For this review, use the dimensioned drawing (mm, ordinates from the lowest corner) and the shaded views. Give positions to 0.01 mm unless a question says otherwise; leave off trailing zeros. Loops run counter-clockwise (first coordinate to the right, second up) from the corner with the lowest first, then second, coordinate; pieces in that order, holes last. Notation, with made-up numbers: M 21.5,80 L 63.5,80 A23 cw 63.5,90 Z; hole C -26,-25.75 d7. An arc over 180 degrees is marked long. Use a Markdown table: item, result. Add a question column.
(1) Add section B-B, the plane y = 30.5. Give the boundary of the cut face in (x, z) (1 decimal), then the cut area to 3 significant figures.
(2) Insertion check: pin 1 Ø5 at (y, z) = (44, 68) entering from -X; pin 2 Ø10 at (y, z) = (14.5, 141.5) entering from -X (1 decimal); pin 3 Ø10 at (y, z) = (6, 19) entering from -X. Each pin has a flat end and moves straight along its axis. Give the tip position at first contact, or say it passes through.
(3) Add section C-C, the plane z = 128. Give the boundary of the cut face in (x, y), then the cut area to 3 significant figures.
(4) For probe 1 along Y at (x, z) = (56.5, 147.5); probe 2 along Y at (x, z) = (107, 66); probe 3 along X at (y, z) = (3, 42.5) (1 decimal), list the stretches that pass through material, from the lowest coordinate up.
(5) Add section D-D, the plane x = 25.5. Give the boundary of the cut face in (y, z) (1 decimal), then the cut area to 3 significant figures.
(6) Draft analysis for pull direction X (two halves, no side actions). For the marked faces 1, 2 and 3, state which applies: pulls with the +X half, pulls with the -X half, needs draft (parallel to the pull), parting line crosses it, or undercut.
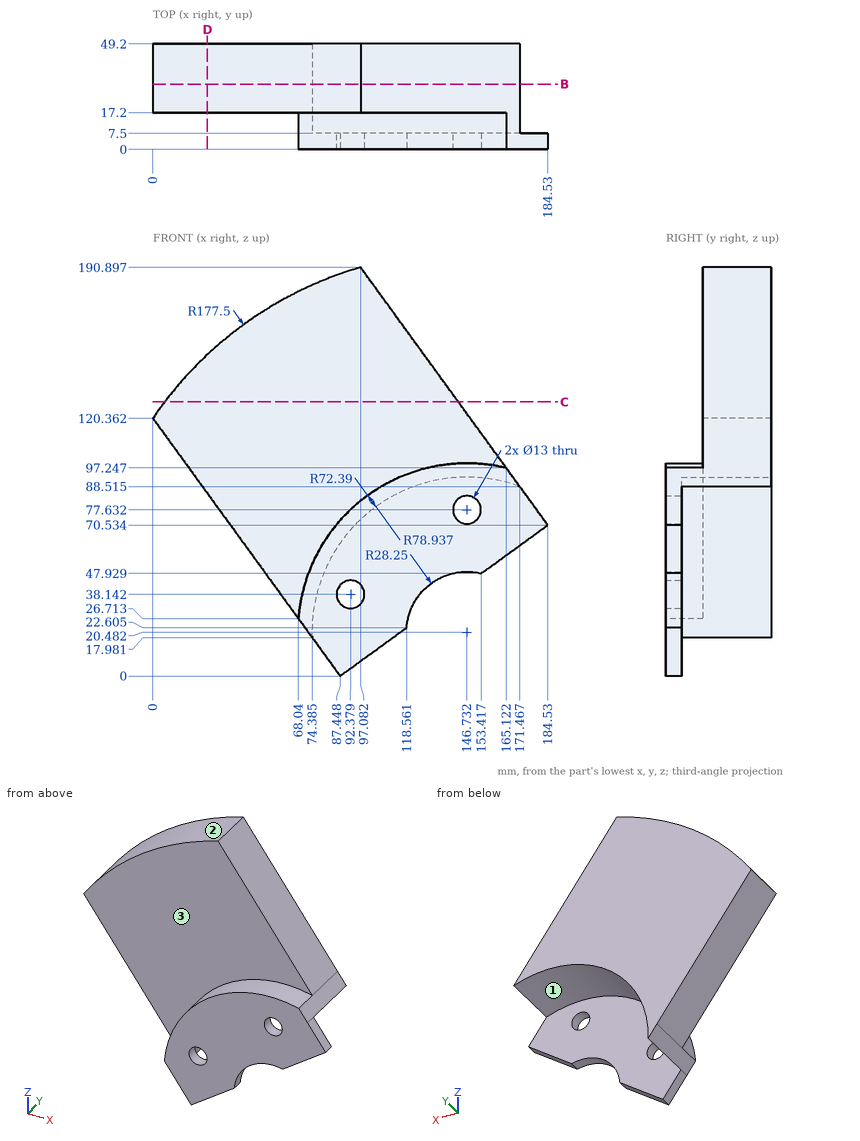
Established:
| question | item | result |
|---|---|---|
| 1 | outline | M 0,120.4 L 74.4,18 A72.4 cw 171.5,88.5 L 97.1,190.9 A177.5 ccw Z |
| 1 | area | 13,300 mm^2 |
| 2 | pin 1 | x = 36.23 |
| 2 | pin 2 | x = 13.1 |
| 2 | pin 3 | x = 70.01 |
| 3 | outline | M 5.5,17.2 L 142.78,17.2 L 142.78,49.2 L 5.5,49.2 Z |
| 3 | area | 4,390 mm^2 |
| 4 | probe 1 | 17.2 to 49.2 |
| 4 | probe 2 | 0 to 7.5 |
| 4 | probe 3 | 70.9 to 87.6, 97.2 to 129 |
| 5 | outline | M 17.2,85.3 L 49.2,85.3 L 49.2,150.1 L 17.2,150.1 Z |
| 5 | area | 2,080 mm^2 |
| 6 | face 1 | undercut |
| 6 | face 2 | pulls with the -X half |
| 6 | face 3 | needs draft |
